For this review, take the finished solid that the model builds, in its own axes (mm). Coordinates: 2 decimals unless noted, no trailing zeros. Write each loop counter-clockwise with the first axis right and the second up, starting at its lowest first coordinate (ties: lowest second). Pieces come first, ordered by that corner, then holes. Notation, with made-up numbers: M 64.25,-24 L 112.25,-24 A12 cw 112.25,-10 Z; hole C 6.5,-21 d9. An arc over 180 degrees is marked long. Return JSON: item names as keys, results as strings.
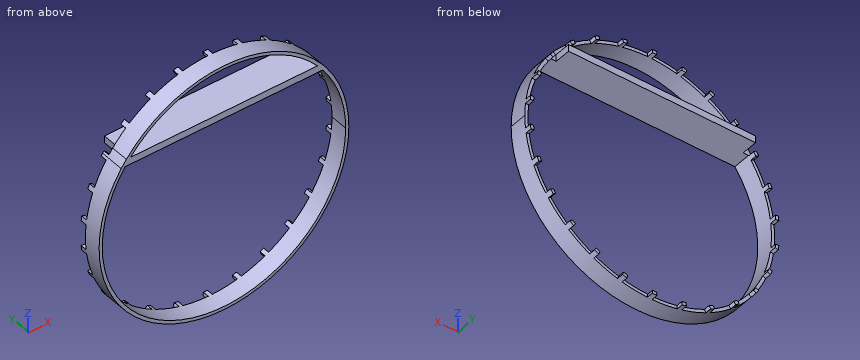
```python
from build123d import *

# Parameters (mm, degrees)
BOSS_EXTRUDE1_DEPTH = 19
SKETCH2_W           = 20
SKETCH2_H           = 11
CUT_EXTRUDE1_DEPTH  = 141.589828935
CIRPATTERN1_COUNT   = 26
SKETCH3_W           = 147.494656174
SKETCH3_H           = 5.46
BOSS_EXTRUDE2_DEPTH = 12.6


with BuildPart() as part:
    # Sketch1 → Boss-Extrude1 (new body)
    with BuildSketch(Plane(origin=(0, 0, 0), x_dir=(1, 0, 0), z_dir=(0, 1, 0))):
        with BuildLine():
            ThreePointArc((76.973491541, -61.46), (79.050100656, -58.765054125), (81.032400927, -56))
            Line((81.032400927, -56), (77.974354758, -56))
            ThreePointArc((77.974354758, -56), (75.90994771, -58.76801714), (73.747328087, -61.46))
            Line((73.747328087, -61.46), (76.973491541, -61.46))
        make_face()
        with BuildLine():
            ThreePointArc((73.747328087, -61.46), (75.90994771, -58.76801714), (77.974354758, -56))
            Line((77.974354758, -56), (-77.974354758, -56))
            ThreePointArc((-77.974354758, -56), (-75.90994771, -58.76801714), (-73.747328087, -61.46))
            Line((-73.747328087, -61.46), (73.747328087, -61.46))
        make_face()
        with BuildLine():
            ThreePointArc((-73.747328087, -61.46), (-75.90994771, -58.76801714), (-77.974354758, -56))
            Line((-77.974354758, -56), (-81.032400927, -56))
            ThreePointArc((-81.032400927, -56), (-79.050100656, -58.765054125), (-76.973491541, -61.46))
            Line((-76.973491541, -61.46), (-73.747328087, -61.46))
        make_face()
        with BuildLine():
            Line((77.974354758, -56), (81.032400927, -56))
            ThreePointArc((81.032400927, -56), (94.031753922, -29.330517458), (98.5, 0))
            ThreePointArc((98.5, 0), (-29.330517458, 94.031753922), (-81.032400927, -56))
            Line((-81.032400927, -56), (-77.974354758, -56))
            ThreePointArc((-77.974354758, -56), (-29.414808713, 91.382542252), (96, 0))
            ThreePointArc((96, 0), (91.382542252, -29.414808713), (77.974354758, -56))
        make_face()
        with BuildLine():
            ThreePointArc((-76.973491541, -61.46), (0, -98.5), (76.973491541, -61.46))
            Line((76.973491541, -61.46), (73.747328087, -61.46))
            ThreePointArc((73.747328087, -61.46), (0, -96), (-73.747328087, -61.46))
            Line((-73.747328087, -61.46), (-76.973491541, -61.46))
        make_face()
    extrude(amount=BOSS_EXTRUDE1_DEPTH)

    # Sketch2 → Cut-Extrude1 (cut, through all)
    with BuildSketch(Plane(origin=(0, 0, 0), x_dir=(0, 0, -1), z_dir=(1, 0, 0))):
        with Locations((0, 19.5)):
            Rectangle(SKETCH2_W, SKETCH2_H)
    cut_extrude1 = extrude(amount=-CUT_EXTRUDE1_DEPTH, mode=Mode.SUBTRACT)

    # CirPattern1: Cut-Extrude1 ×26 about axis
    cirpattern1_axis = Axis((0, 0, 0), (0, 1, 0))
    for i in range(1, CIRPATTERN1_COUNT):
        add(cut_extrude1.rotate(cirpattern1_axis, i * 360 / CIRPATTERN1_COUNT), mode=Mode.SUBTRACT)

    # Sketch3 → Boss-Extrude2 (add)
    with BuildSketch(Plane(origin=(0, 14, 0), x_dir=(1, 0, 0), z_dir=(0, 1, 0))):
        with Locations((0, -58.73)):
            Rectangle(SKETCH3_W, SKETCH3_H)
    extrude(amount=BOSS_EXTRUDE2_DEPTH)


solid = part.part
```
1. We need section A-A (y = 4.5). State the section outline as (x, z) points.
Checks:
{"outline": "C 0,0 d197; hole M -77.97,56 A96 ccw long 77.97,56 Z; hole M -73.75,61.46 L 73.75,61.46 A96 ccw Z"}
2. Wall thickness on L1, parallel to Z at x = 0, y = 15.25; L2, parallel to X at y = 7, z = 0; L3, parallel to Z at x = 26, y = 9.5: over which ranges is each line inside the solid? List them lowest first. Write a range as from..to.
Checks:
{"L1": "-98.5..-96, 56..61.46, 96..98.5", "L2": "-98.5..-96, 96..98.5", "L3": "-95.01..-92.41, 56..61.46, 92.41..95.01"}
3. Clearance check with flat-ended pins moving along their axes: pin 1 Ø1.4 at (x, z) = (-96.5, 11) entering from +Y; pin 2 Ø6.5 at (x, z) = (-53.5, 80.5) entering from +Y; pin 3 Ø1 at (x, y) = (9.5, 12.5) entering from +Z; pin 4 Ø3.5 at (x, z) = (-83.5, 42.5) entering from +Y. State where each tip first meets the part, or that it passes through.
Checks:
{"pin 1": "y = 19", "pin 2": "y = 14", "pin 3": "z = 98.09", "pin 4": "through"}
4. We need section D-D (z = 25.5). State the section outline as (x, y) points, plus the area to 3 significant figures.
Checks:
{"outline": "M -95.14,0 L -92.55,0 L -92.55,14 L -95.14,14 Z; M 92.55,0 L 95.14,0 L 95.14,14 L 92.55,14 Z", "area": "72.5 mm2"}
5. We need section C-C (y = 16.5). Give the number of separate pieces and of enclosed holes in the cut face, plus the area to 3 significant figures.
Checks:
{"separate pieces": "27", "enclosed holes": "0", "area": "1,030 mm2"}
6. We need section B-B (z = -44). State the section outline as (x, y) points.
Checks:
{"outline": "M -88.13,0 L -85.32,0 L -85.32,14 L -88.13,14 Z; M 85.32,0 L 88.13,0 L 88.13,14 L 85.32,14 Z"}
